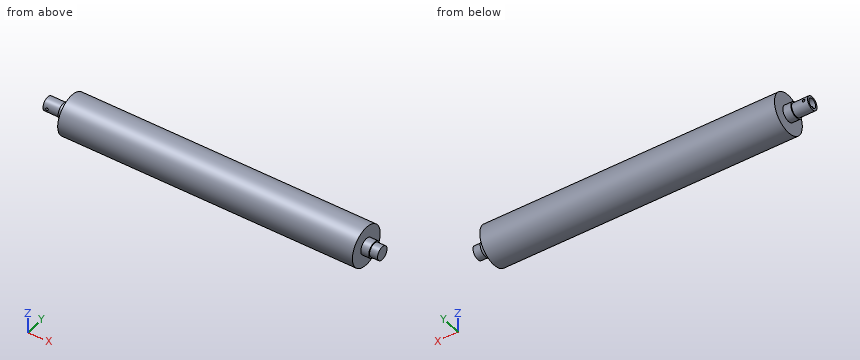
from build123d import *

# Parameters (mm, degrees)
HOLE_WIZARD_M4_1_D     = 3.3
HOLE_WIZARD_M4_1_DEPTH = 20
HOLE_WIZARD_M4_1_TIP   = 0.991420021
MM_CLEARANCE_1_D       = 12.1
MM_CLEARANCE_1_DEPTH   = 12
MM_CLEARANCE_1_TIP     = 3.635206745


with BuildPart() as part:
    # 草图2 → 旋转1 (revolve)
    with BuildSketch(Plane.XY):
        Polygon((354.507854502, 10), (344.507854502, 10), (344.507854502, 25), (-25.492145498, 25), (-25.492145498, 10), (-35.492145498, 10), (-35.492145498, 8.5), (-45.492145498, 8.5), (-55.492145498, 8.5), (-55.492145498, 0), (-39.793794406, 0), (364.507854502, 0), (364.507854502, 8.5), (354.507854502, 8.5), align=None)
    revolve(axis=Axis((-62.705882353, 0, 0), (1, 0, 0)))

    # M4 螺纹孔1
    with Locations(Plane(origin=(0, 8.5, 0), x_dir=(1, 0, 0), z_dir=(0, 1, 0))):
        with Locations((-50.492145498, 0)):
            Hole(HOLE_WIZARD_M4_1_D / 2, depth=HOLE_WIZARD_M4_1_DEPTH)
            with Locations((0, 0, -(HOLE_WIZARD_M4_1_DEPTH + HOLE_WIZARD_M4_1_TIP / 2))):  # 118° drill point
                Cone(0, HOLE_WIZARD_M4_1_D / 2, HOLE_WIZARD_M4_1_TIP, mode=Mode.SUBTRACT)

    # 大小mm Clearance 暗销孔1
    with Locations(Plane.ZY.offset(55.492145498)):
        with Locations((0, 0)):
            Hole(MM_CLEARANCE_1_D / 2, depth=MM_CLEARANCE_1_DEPTH)
            with Locations((0, 0, -(MM_CLEARANCE_1_DEPTH + MM_CLEARANCE_1_TIP / 2))):  # 118° drill point
                Cone(0, MM_CLEARANCE_1_D / 2, MM_CLEARANCE_1_TIP, mode=Mode.SUBTRACT)


solid = part.part
Geometry check sheet. Reference: the model listing, model coordinates, mm. Round coordinates to 2 decimals unless told otherwise and drop trailing zeros. Order: outer loops, then holes, each group sorted by start corner. A loop starts at its lowest first (then second) coordinate and runs counter-clockwise, first axis right, second up. Notation, with made-up numbers: M 66.5,36.25 L 107.5,36.25 A28 ccw 107.5,62.25 Z; hole C -14.5,54 d11. An arc over 180 degrees is marked long. Answer in a Markdown table with one row per item.
(1) Go/stop test with flat-tipped pins: P1, Ø5, axis at y = -18, z = 6, coming from the +X side; P2, Ø12, axis at y = 18, z = -17.5, coming from the -X side; P3, Ø4, axis at y = 5.5, z = 0, coming from the -X side; P4, Ø1, axis at x = 206, y = 1.5, coming from the -Z side. Record where each tip stops, or that it passes through.
Responses:
| item | result |
|---|---|
| P1 | stops at x = 344.51 |
| P2 | stops at x = -25.49 |
| P3 | stops at x = -55.49 |
| P4 | stops at z = -24.98 |
(2) Scan lines: probe 1 along Z at (x, y) = (-51.5, 0); probe 2 along X at (y, z) = (-8, -3.5). Record each from-to range of solid material in increasing order. Write a range as from..to.
Responses:
| item | result |
|---|---|
| probe 1 | z = -8.5..-6.05, 6.05..8.5 |
| probe 2 | x = -35.49..354.51 |
(3) Sectioned sample at C-C, the plane z = 19. Record the cut outline in (x, y).
Responses:
| item | result |
|---|---|
| outline | M -25.49,-16.25 L 344.51,-16.25 L 344.51,16.25 L -25.49,16.25 Z |
(4) Sectioned sample at A-A, the plane x = 0.5. Record the cut outline in (y, z), and give its area (3 significant figures).
Responses:
| item | result |
|---|---|
| outline | C 0,0 d50 |
| area | 1,960 mm² |
(5) Sectioned sample at B-B, the plane y = 13.5. Record the cut outline in (x, z).
Responses:
| item | result |
|---|---|
| outline | M -25.49,-21.04 L 344.51,-21.04 L 344.51,21.04 L -25.49,21.04 Z |
